from build123d import *

# Parameters (mm, degrees)
SKETCH_1_R      = 2
EXTRUDE_1_DEPTH = 2.8


with BuildPart() as part:
    # 草图1 → 凸台-拉伸1 (new body)
    with BuildSketch(Plane.XY):
        Polygon((0, 3.695041723), (-3.2, 1.847520861), (-3.2, -1.847520861), (0, -3.695041723), (3.2, -1.847520861), (3.2, 1.847520861), align=None)
        Circle(SKETCH_1_R, mode=Mode.SUBTRACT)
    extrude(amount=EXTRUDE_1_DEPTH)

    # 草图2 → 切除-旋转1 (revolve, cut)
    with BuildSketch(Plane(origin=(0, 0, 0), x_dir=(0, 0, -1), z_dir=(1, 0, 0)), mode=Mode.PRIVATE) as cut_revolve_1_sk:
        Polygon((-2.364617701, 3.695041723), (-2.8, 3.026797752), (-2.8, 3.695041723), align=None)
    cut_revolve_1 = revolve(cut_revolve_1_sk.sketch.rotate(Axis((0, 0, 2.8), (0, 0, -1)), 300.000000046), axis=Axis((0, 0, 2.8), (0, 0, -1)), mode=Mode.SUBTRACT)

    # 镜向1: 切除-旋转1 across plane
    add(cut_revolve_1.mirror(Plane(origin=(0, 0, 1.4), x_dir=(1, 0, 0), z_dir=(0, 0, -1))), mode=Mode.SUBTRACT)


solid = part.part
Design review of the part built by this model. Coordinates are the model's own, in mm. Coordinates: 2 decimals unless noted, no trailing zeros. Write each loop counter-clockwise with the first axis right and the second up, starting at its lowest first coordinate (ties: lowest second). Pieces come first, ordered by that corner, then holes. Notation, with made-up numbers: (66, 19.25) -> (122, 19.25) arc R18 cw to (122, 32.25) -> close; hole circle Ø7 at (56, 43). An arc over 180 degrees is marked (long way). Write each question's results on one line, items separated by ' | '. Start each with the question number.
(1) The part is to be moulded in two halves that separate along Y. For faces 1 (the face through (1, -2, 2.8)), 2 (the face through (-1.578, 2.784, 1.382)), 3 (the face through (0, -2, 1)), say which applies: pulls with the +Y half, pulls with the -Y half, needs draft (parallel to the pull), parting line crosses it, or undercut.
(2) For line 1 along X through (y, z) = (-1.25, 0.35); line 2 along X through (y, z) = (-1, 1.1); line 3 along Y through (x, z) = (2.5, 0.95), list the stretches that pass through material, from the lowest coordinate up. Write a range as from..to.
(3) Take a section at B-B on z = 0.9. Write out the cut boundary in (x, y), and give its area (3 significant figures).
(4) Take a section at A-A on y = 0. Write out the cut boundary in (x, z), and give its area (3 significant figures).
Results found:
1) face 1: needs draft | face 2: pulls with the +Y half | face 3: undercut
2) line 1: x = -3.2..-1.56, 1.56..3.2 | line 2: x = -3.2..-1.73, 1.73..3.2 | line 3: y = -2.25..2.25
3) outline: (-3.2, -1.85) -> (0, -3.7) -> (3.2, -1.85) -> (3.2, 1.85) -> (0, 3.7) -> (-3.2, 1.85) -> close; hole circle Ø4 at (0, 0) | area: 22.9 mm2
4) outline: (-3.2, 0.11) -> (-3.03, 0) -> (-2, 0) -> (-2, 2.8) -> (-3.03, 2.8) -> (-3.2, 2.69) -> close; (2, 0) -> (3.03, 0) -> (3.2, 0.11) -> (3.2, 2.69) -> (3.03, 2.8) -> (2, 2.8) -> close | area: 6.68 mm2
